```python
from build123d import *

# Parameters (mm, degrees)
F0_W     = 60
F0_H     = 60
F1_DEPTH = 5
F2_W     = 58
F2_H     = 58
F3_DEPTH = 2.5
F4_W     = 1
F4_H     = 58
F5_DEPTH = 2.5


with BuildPart() as f1:
    # F0 (on Top) → F1 (new body)
    with BuildSketch(Plane.XY):
        with Locations((30, 30)):
            Rectangle(F0_W, F0_H)
    extrude(amount=F1_DEPTH)

    # F2 (on face) → F3 (cut)
    with BuildSketch(Plane.XY.offset(5)):
        with Locations((30, 30)):
            Rectangle(F2_W, F2_H)
    extrude(amount=-F3_DEPTH, mode=Mode.SUBTRACT)

    # F4 (on face) → F5 (join)
    with BuildSketch(Plane.XY.offset(2.5)):
        with Locations((2.5, 30)):
            Rectangle(F4_W, F4_H)
        with Locations((4.5, 30)):
            Rectangle(F4_W, F4_H)
        with Locations((6.5, 30)):
            Rectangle(F4_W, F4_H)
        with Locations((8.5, 30)):
            Rectangle(F4_W, F4_H)
        with Locations((10.5, 30)):
            Rectangle(F4_W, F4_H)
        with Locations((12.5, 30)):
            Rectangle(F4_W, F4_H)
        with Locations((14.5, 30)):
            Rectangle(F4_W, F4_H)
        with Locations((16.5, 30)):
            Rectangle(F4_W, F4_H)
        with Locations((18.5, 30)):
            Rectangle(F4_W, F4_H)
        with Locations((20.5, 30)):
            Rectangle(F4_W, F4_H)
    extrude(amount=F5_DEPTH)


solid = f1.part
```
Check sheet for the modelled part. Datum: model origin and axes. Units: mm. Round coordinates to 2 decimals unless told otherwise and drop trailing zeros. Order: outer loops, then holes, each group sorted by start corner. A loop starts at its lowest first (then second) coordinate and runs counter-clockwise, first axis right, second up.
1) Go/stop test with a flat-tipped pin: pin 1 Ø11.5 at (x, y) = (48.5, 21.5) entering from +Z. Record where the tip stops, or that it passes through.
2) Section check B-B (z = 4). Give the number of separate pieces and of enclosed holes in the cut face, and give its area (3 significant figures).
3) Section check A-A (x = 55.5). Record the boundary of the cut face in (y, z), and give its area (3 significant figures).
4) Mould release check, pull along X, two halves, no side actions. Record for faces 1 (the flat face through (40, 59, 4)), 2 (the flat face through (60, 30, 2)), 3 (the flat face through (0, 30, 2)): +X half, -X half, draft (parallel to the pull), parting line (faces both ways), or undercut.
5) Scan lines: line 1 (Y direction, x = 32, z = 4.7); line 2 (Z direction, x = 24, y = 29). Record each from-to range of solid material in increasing order.
Result:
1. pin 1: stops at z = 2.5
2. separate pieces: 1
2. enclosed holes: 11
2. area: 816 mm2
3. outline: (0, 0) - (60, 0) - (60, 5) - (59, 5) - (59, 2.5) - (1, 2.5) - (1, 5) - (0, 5) - close
3. area: 155 mm2
4. face 1: undercut
4. face 2: +X half
4. face 3: -X half
5. line 1: y = 0 to 1, 59 to 60
5. line 2: z = 0 to 2.5
